from build123d import *

# Parameters (mm, degrees)
F0_W     = 152.4
F0_H     = 50.8
F2_DEPTH = 25.4
F1_W     = 127
F1_H     = 38.1
F3_DEPTH = 25.4
F4_W     = 61.2871721387
F4_H     = 12.1671258756
F5_DEPTH = 78.74
F6_W     = 73.1669291854
F6_H     = 12.5516466796
F7_DEPTH = 60.96


with BuildPart() as f2:
    # F0 (on Front) → F2 (new body)
    with BuildSketch(Plane.XZ):
        with Locations((2.4711750448, -43.9968049534)):
            Rectangle(F0_W, F0_H)
    extrude(amount=F2_DEPTH)

    # F1 (on Front) → F3 (join)
    with BuildSketch(Plane.XZ):
        with Locations((-10.2288249552, 0.4531950466)):
            Rectangle(F1_W, F1_H)
    extrude(amount=F3_DEPTH)

    # F4 (on Right) → F5 (join)
    with BuildSketch(Plane.YZ):
        with Locations((30.6435860693, -63.3132420157)):
            Rectangle(F4_W, F4_H)
    extrude(amount=F5_DEPTH)

    # F6 (on Front) → F7 (join)
    with BuildSketch(Plane.XZ):
        with Locations((-36.5834645927, -63.2174480706)):
            Rectangle(F6_W, F6_H)
    extrude(amount=-F7_DEPTH)


solid = f2.part
Can you work these out from the model? Positions are in its coordinate system, mm. A direction names the side the tool comes from. Coordinates: 2 decimals unless noted, no trailing zeros. Loops run counter-clockwise (first coordinate to the right, second up) from the corner with the lowest first, then second, coordinate; pieces in that order, holes last. Notation, with made-up numbers: (-31.5, -15.75) - (-18.5, -15.75) arc R28 ccw to (-18.5, 17.25) - close; hole circle Ø4 at (22.5, 31.5). An arc over 180 degrees is marked (long way). Answer as a JSON object with one key per item and string values. Group by question number.
Item 1: If I drill on L1, parallel to Z at x = 63, y = 20.5; L2, parallel to Y at x = 43, z = -43; L3, parallel to Z at x = -43.5, y = 30, over which ranges is the centre line in solid material (lowest first)? Write a range as from..to.
Item 2: For pin 1 (2 mm diameter, centred on x = 62.5, z = -43, fed in from +Y); pin 2 (18.5 mm diameter, centred on x = 33, y = 22, fed in from +Z); pin 3 (12.5 mm diameter, centred on y = -18.5, z = -33, fed in from +X), each with a flat end and sliding along its axis, tell me the tip position at first contact or that it passes through.
Item 3: If we section it at A-A (x = -15): List the corners of the cut face in (y, z) for me, plus the area to 3 significant figures.
Item 4: On a 3-axis mill with a long thin cutter (end or side, diameter ignored), from which of +Z, -Z, +X, -X, +Y, -Y can I reach the whole of each face in a straight line? I mean faces 1 (the face through (39, 30, -57.23)), 2 (the face through (53.271, -13, 0)), 3 (the face through (-37, 60.96, -63)). Say none if no direction works.
Item 5: If we section it at C-C (z = -51): List the corners of the cut face in (x, y) for me.
Item 6: If we section it at B-B (y = 21): List the corners of the cut face in (x, z) for me, plus the area to 3 significant figures.
Item 7: If we section it at D-D (x = 39.5): List the corners of the cut face in (y, z) for me, plus the area to 3 significant figures.
Returned:
{
 "1": {"L1": "z = -69.4..-57.23", "L2": "y = -25.4..0", "L3": "z = -69.49..-56.94"},
 "2": {"pin 1": "stops at y = 0", "pin 2": "stops at z = -57.23", "pin 3": "stops at x = 78.67"},
 "3": {"outline": "(-25.4, -69.4) - (0, -69.4) - (0, -69.49) - (60.96, -69.49) - (60.96, -56.94) - (0, -56.94) - (0, 19.5) - (-25.4, 19.5) - close", "area": "3,020 mm²"},
 "4": {"face 1": "+Z, +X, +Y", "face 2": "+Z, +X, +Y, -Y", "face 3": "+Z, -Z, -X, +Y"},
 "5": {"outline": "(-73.73, -25.4) - (78.67, -25.4) - (78.67, 0) - (-73.73, 0) - close"},
 "6": {"outline": "(-73.17, -69.49) - (0, -69.49) - (0, -69.4) - (78.74, -69.4) - (78.74, -57.23) - (0, -57.23) - (0, -56.94) - (-73.17, -56.94) - close", "area": "1,880 mm²"},
 "7": {"outline": "(-25.4, -69.4) - (61.29, -69.4) - (61.29, -57.23) - (0, -57.23) - (0, 19.5) - (-25.4, 19.5) - close", "area": "3,000 mm²"}
}
